Could you check a few things on this drawing? It's one solid part, dimensions in mm from its lowest x, y, z. A direction names the side the tool comes from. Coordinates: 2 decimals unless noted, no trailing zeros. Order: outer loops, then holes, each group sorted by start corner. A loop starts at its lowest first (then second) coordinate and runs counter-clockwise, first axis right, second up. Notation, with made-up numbers: (-23, 86) -> (0, 86) arc R7 ccw to (0, 91) -> close; hole circle Ø4 at (-36.5, 20.5). An arc over 180 degrees is marked (long way). Use a Markdown table: item, result. Add a question column.
1. Suppose I cut it at D-D, the plane z = 15.5. List the corners of the cut face in (x, y) for me.
2. If I drill on line 1 along Y through (x, z) = (17.5, 3.5); line 2 along Z through (x, y) = (18, 28); line 3 along X through (y, z) = (17.5, 9), over which ranges is the centre line in solid material (lowest first)? Write a range as from..to.
3. For the marked faces 4, 5, 6, 7 and 8, which set-ups out of +Z, -Z, +X, -X, +Y, -Y let a thin tool reach every point of the face, with its end or its side?
4. We'd pull the mould along Z, two halves only. Please class the marked faces 1, 2 and 3: pulls with the +Z half, pulls with the -Z half, needs draft (parallel to the pull), parting line crosses it, or undercut.
5. For pin 1 Ø7 at (x, y) = (13, 17) entering from -Z; pin 2 Ø7.5 at (x, y) = (17.5, 17.5) entering from -Z; pin 3 Ø1.7 at (y, z) = (17, 10) entering from -X; pin 4 Ø1.7 at (y, z) = (16, 9.5) entering from +X, each with a flat end and sliding along its axis, tell me the tip position at first contact or that it passes through.
6. Suppose I cut it at B-B, the plane y = 17.5. List the corners of the cut face in (x, z) for me, then the cut area to 3 significant figures.
7. Suppose I cut it at A-A, the plane z = 7.25. List the corners of the cut face in (x, y) for me, then the cut area to 3 significant figures.
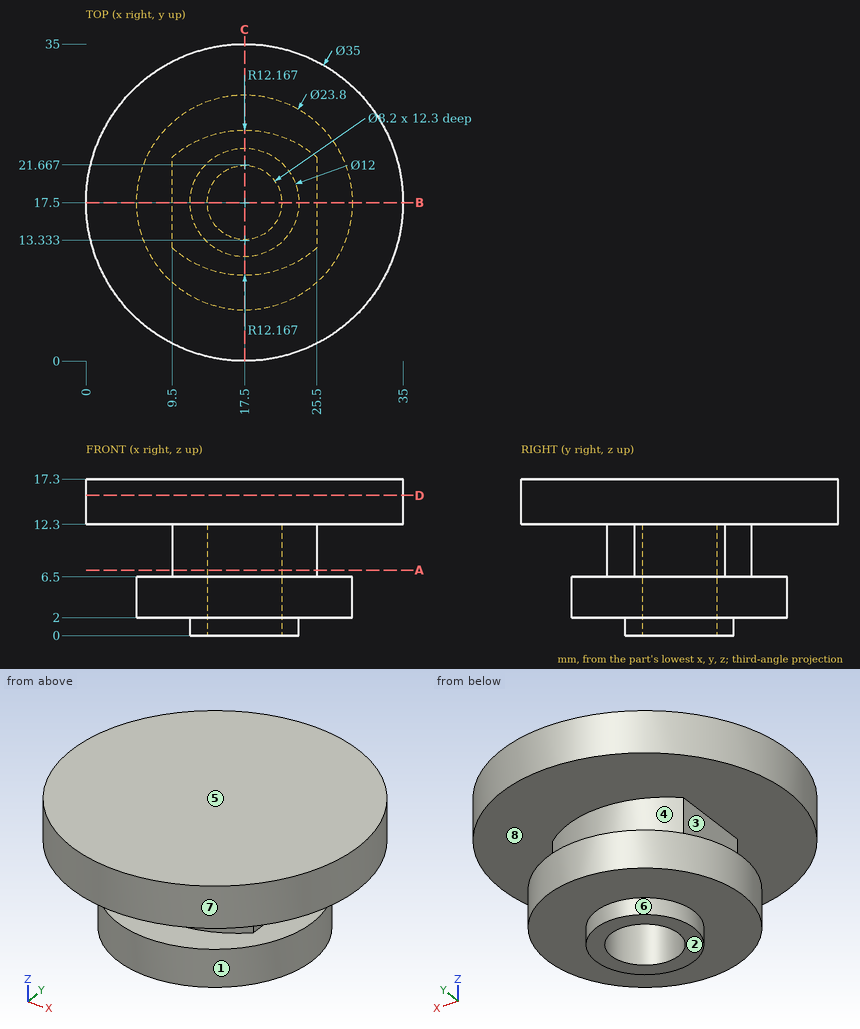
Worked out:
| question | item | result |
|---|---|---|
| 1 | outline | circle Ø35 at (17.5, 17.5) |
| 2 | line 1 | y = 5.6..13.4, 21.6..29.4 |
| 2 | line 2 | z = 2..6.5, 12.3..17.3 |
| 2 | line 3 | x = 9.5..13.4, 21.6..25.5 |
| 3 | face 4 | +Y |
| 3 | face 5 | +Z, +X, -X, +Y, -Y |
| 3 | face 6 | -Z |
| 3 | face 7 | +Z, -Z |
| 3 | face 8 | none |
| 4 | face 1 | needs draft |
| 4 | face 2 | pulls with the -Z half |
| 4 | face 3 | undercut |
| 5 | pin 1 | stops at z = 0 |
| 5 | pin 2 | stops at z = 12.3 |
| 5 | pin 3 | stops at x = 9.5 |
| 5 | pin 4 | stops at x = 25.5 |
| 6 | outline | (0, 12.3) -> (9.5, 12.3) -> (9.5, 6.5) -> (5.6, 6.5) -> (5.6, 2) -> (11.5, 2) -> (11.5, 0) -> (13.4, 0) -> (13.4, 12.3) -> (21.6, 12.3) -> (21.6, 0) -> (23.5, 0) -> (23.5, 2) -> (29.4, 2) -> (29.4, 6.5) -> (25.5, 6.5) -> (25.5, 12.3) -> (35, 12.3) -> (35, 17.3) -> (0, 17.3) -> close |
| 6 | area | 298 mm² |
| 7 | outline | (9.5, 12.5) arc R12.17 ccw to (25.5, 12.5) -> (25.5, 22.5) arc R12.17 ccw to (9.5, 22.5) -> close; hole circle Ø8.2 at (17.5, 17.5) |
| 7 | area | 173 mm² |
